The model under review builds one solid part; all positions refer to its coordinate system, in mm. A direction names the side the tool comes from. Round coordinates to 2 decimals unless told otherwise and drop trailing zeros. Order: outer loops, then holes, each group sorted by start corner. A loop starts at its lowest first (then second) coordinate and runs counter-clockwise, first axis right, second up. Notation, with made-up numbers: (88.25, 44.5) -> (94.25, 44.5) arc R23 cw to (94.25, 65.5) -> close; hole circle Ø10 at (73.25, 15). An arc over 180 degrees is marked (long way). Put each result on its own line as item: value. Start each with the question number.
from build123d import *

# Parameters (mm, degrees)
F0_W     = 170.18
F0_H     = 174.625
F1_DEPTH = 1.5875
F2_W     = 170.18
F2_H     = 174.625
F2_W_2   = 167.005
F2_H_2   = 171.45
F3_DEPTH = 22.5425
F5_DEPTH = 0.79375


with BuildPart() as f1:
    # F0 (on Top) → F1 (new body)
    with BuildSketch(Plane.XY):
        Rectangle(F0_W, F0_H)
    extrude(amount=F1_DEPTH)

    # F2 (on face) → F3 (join)
    with BuildSketch(Plane.XY.offset(1.5875)):
        Rectangle(F2_W, F2_H)
        Rectangle(F2_W_2, F2_H_2, mode=Mode.SUBTRACT)
    extrude(amount=F3_DEPTH)

    # F4 (on Right) → F5 (join, symmetric)
    with BuildSketch(Plane.YZ):
        with BuildLine():
            Line((-87.3125, 7.356259), (-87.3125, 21.853741))
            ThreePointArc((-87.3125, 21.853741), (-92.583, 14.605), (-87.3125, 7.356259))
        make_face()
    extrude(amount=F5_DEPTH, both=True)


solid = f1.part
Q1. Clearance check with flat-ended pins moving along their axes: pin 1 Ø1.5 at (x, y) = (-40, -71) entering from +Z; pin 2 Ø10 at (x, z) = (-4.5, 7.5) entering from -Y; pin 3 Ø12 at (x, z) = (-12, 10.5) entering from -Y. State where each tip first meets the part, or that it passes through.
Q2. Take a section at C-C on y = 68. Give the boundary of the cut face in (x, z).
Q3. Take a section at A-A on z = 5.25. Give the boundary of the cut face in (x, y) (1 decimal), and give its area (3 significant figures).
Q4. Wall thickness on probe 1 along X at (y, z) = (-53, 9); probe 2 along Y at (x, z) = (66.5, 15) (1 decimal); probe 3 along Z at (x, y) = (-27.5, -66): over which ranges is each line inside the solid? List them lowest first. Write a range as [from, to].
Q5. Take a section at D-D on z = 16.5. Give the boundary of the cut face in (x, y) (1 decimal).
Q6. Take a section at B-B on x = -11. Give the boundary of the cut face in (y, z) (1 decimal), and give its area (3 significant figures).
Q7. Draft analysis for pull direction Y (two halves, no side actions). For faces 6 (the face through (-1, 1, 0)), 7 (the face through (-83.502, -1, 13)), 8 (the face through (-1, 87.312, 12)), state which applies: +Y half, -Y half, draft (parallel to the pull), parting line (faces both ways), or undercut.
Q8. For faces 1 (the face through (0.794, -89, 15)), 2 (the face through (-0.794, -89, 15)), 3 (the face through (-85.09, -1, 12)), 4 (the face through (85.09, -1, 12)), 5 (the face through (-1, 1, 1.588)), list the 3-axis set-ups (+Z, -Z, +X, -X, +Y, -Y) from which the entire face can be reached by the end or side of a thin tool; tool diameter is ignored.
Calculated:
1. pin 1: stops at z = 1.59
1. pin 2: stops at y = -91.6
1. pin 3: stops at y = -87.31
2. outline: (-85.09, 0) -> (85.09, 0) -> (85.09, 24.13) -> (83.5, 24.13) -> (83.5, 1.59) -> (-83.5, 1.59) -> (-83.5, 24.13) -> (-85.09, 24.13) -> close
3. outline: (-85.1, -87.3) -> (85.1, -87.3) -> (85.1, 87.3) -> (-85.1, 87.3) -> close; hole (-83.5, -85.7) -> (83.5, -85.7) -> (83.5, 85.7) -> (-83.5, 85.7) -> close
3. area: 1,080 mm²
4. probe 1: x = [-85.09, -83.5], [83.5, 85.09]
4. probe 2: y = [-87.3, -85.7], [85.7, 87.3]
4. probe 3: z = [0, 1.59]
5. outline: (-85.1, -87.3) -> (-0.8, -87.3) -> (-0.8, -92.3) -> (0.8, -92.3) -> (0.8, -87.3) -> (85.1, -87.3) -> (85.1, 87.3) -> (-85.1, 87.3) -> close; hole (-83.5, -85.7) -> (83.5, -85.7) -> (83.5, 85.7) -> (-83.5, 85.7) -> close
6. outline: (-87.3, 0) -> (87.3, 0) -> (87.3, 24.1) -> (85.7, 24.1) -> (85.7, 1.6) -> (-85.7, 1.6) -> (-85.7, 24.1) -> (-87.3, 24.1) -> close
6. area: 349 mm²
7. face 6: draft
7. face 7: undercut
7. face 8: +Y half
8. face 1: +Z, -Z, +X, -Y
8. face 2: +Z, -Z, -X, -Y
8. face 3: +Z, -Z, -X, +Y, -Y
8. face 4: +Z, -Z, +X, +Y, -Y
8. face 5: +Z
